Check sheet for the modelled part. Datum: model origin and axes. Units: mm. A direction names the side the tool comes from. Round coordinates to 2 decimals unless told otherwise and drop trailing zeros. Write each loop counter-clockwise with the first axis right and the second up, starting at its lowest first coordinate (ties: lowest second). Pieces come first, ordered by that corner, then holes. Notation, with made-up numbers: (-36.75, -39.5) -> (6.25, -39.5) arc R18 cw to (6.25, -8.5) -> close; hole circle Ø2 at (37, 55.5). An arc over 180 degrees is marked (long way). Put each result on its own line as item: value. Start each with the question number.
from build123d import *

# Parameters (mm, degrees)
F0_R     = 12.7
F1_DEPTH = 7
F2_R     = 6.5
F3_DEPTH = 10
F4_R     = 4
F5_DEPTH = 10.001
F6_DEPTH = 7.001
F8_D     = 5
F8_DEPTH = 12.701


with BuildPart() as f1:
    # F0 (on Front) → F1 (new body)
    with BuildSketch(Plane.XZ):
        Circle(F0_R)
    extrude(amount=F1_DEPTH)

    # F2 (on Front) → F3 (join)
    with BuildSketch(Plane.XZ):
        Circle(F2_R)
    extrude(amount=-F3_DEPTH)

    # F4 (on Front) → F5 (cut, through all)
    with BuildSketch(Plane.XZ):
        Circle(F4_R)
    extrude(amount=-F5_DEPTH, mode=Mode.SUBTRACT)

    # F6 (cut, through all): a face of the model
    f6_faces = [f1.faces().sort_by_distance(p)[0] for p in [
        (0, 0, 0),
    ]]
    extrude(f6_faces, amount=-F6_DEPTH, mode=Mode.SUBTRACT)

    # F8 (through all, one way)
    with BuildSketch(Plane.XY):
        with Locations((0, 5)):
            Circle(F8_D / 2)
    extrude(amount=-F8_DEPTH, mode=Mode.SUBTRACT)


solid = f1.part
1. Access from +Z, -Z, +X, -X, +Y, -Y to the whole of each face (thin tool, end or side, straight path). Record for faces 4 (the flat face through (-6, 0, 3)), 5 (the flat face through (-3, -7, 3)).
2. Section check B-B, the plane z = 0. Enter the section's corners in (x, y), then the cut area to 3 significant figures.
3. Section check C-C, the plane y = -3.25. Enter the section's corners in (x, z), then the cut area to 3 significant figures.
4. Material ranges on L1, parallel to Z at x = 0, y = -2.75; L2, parallel to Y at x = 0, z = -4.45; L3, parallel to Y at x = 0.5, z = -8, recorded low to high. Write a range as [from, to].
5. Draft check along Y on faces 1 (the cylindrical face through (-2.75, -3.45, -12.4)), 2 (the flat face through (3, 10, 3)), 3 (the cylindrical face through (2.385, 5.751, -4.789)). Enter one of: released by +Y, released by -Y, zero draft, split by the parting line, or undercut.
6. Section check A-A, the plane x = 0. Enter the section's corners in (y, z).
7. Section check D-D, the plane z = 3. Enter the section's corners in (x, y), then the cut area to 3 significant figures.
8. Gauge pin test, flat ends, axial feed: P1, Ø4.5, axis at x = 0, y = 5, coming from the -Z side; P2, Ø5, axis at y = 3, z = 7.5, coming from the +X side; P3, Ø2, axis at y = 5, z = 3.5, coming from the -X side. Record the tip position at first contact, or that the pin passes through.
Reply:
1. face 4: +Y
1. face 5: +Z, -Z, +X, -X, -Y
2. outline: (-12.7, -7) -> (-4, -7) -> (-4, 10) -> (-6.5, 10) -> (-6.5, 0) -> (-12.7, 0) -> close; (4, -7) -> (12.7, -7) -> (12.7, 0) -> (6.5, 0) -> (6.5, 10) -> (4, 10) -> close
2. area: 172 mm2
3. outline: circle Ø25.4 at (0, 0); hole circle Ø8 at (0, 0)
3. area: 456 mm2
4. L1: z = [-12.7, -4], [4, 12.7]
4. L2: y = [-7, 2.5], [7.5, 10]
4. L3: y = [-7, 0]
5. face 1: zero draft
5. face 2: released by +Y
5. face 3: undercut
6. outline: (-7, -12.7) -> (0, -12.7) -> (0, -6.5) -> (2.5, -6.5) -> (2.5, -4) -> (-7, -4) -> close; (-7, 4) -> (10, 4) -> (10, 6.5) -> (0, 6.5) -> (0, 12.7) -> (-7, 12.7) -> close; (7.5, -6.5) -> (10, -6.5) -> (10, -4) -> (7.5, -4) -> close
7. outline: (-12.34, -7) -> (-2.65, -7) -> (-2.65, 10) -> (-5.77, 10) -> (-5.77, 0) -> (-12.34, 0) -> close; (2.65, -7) -> (12.34, -7) -> (12.34, 0) -> (5.77, 0) -> (5.77, 10) -> (2.65, 10) -> close
7. area: 198 mm2
8. P1: stops at z = 3.31
8. P2: stops at x = 4.15
8. P3: stops at x = -6
